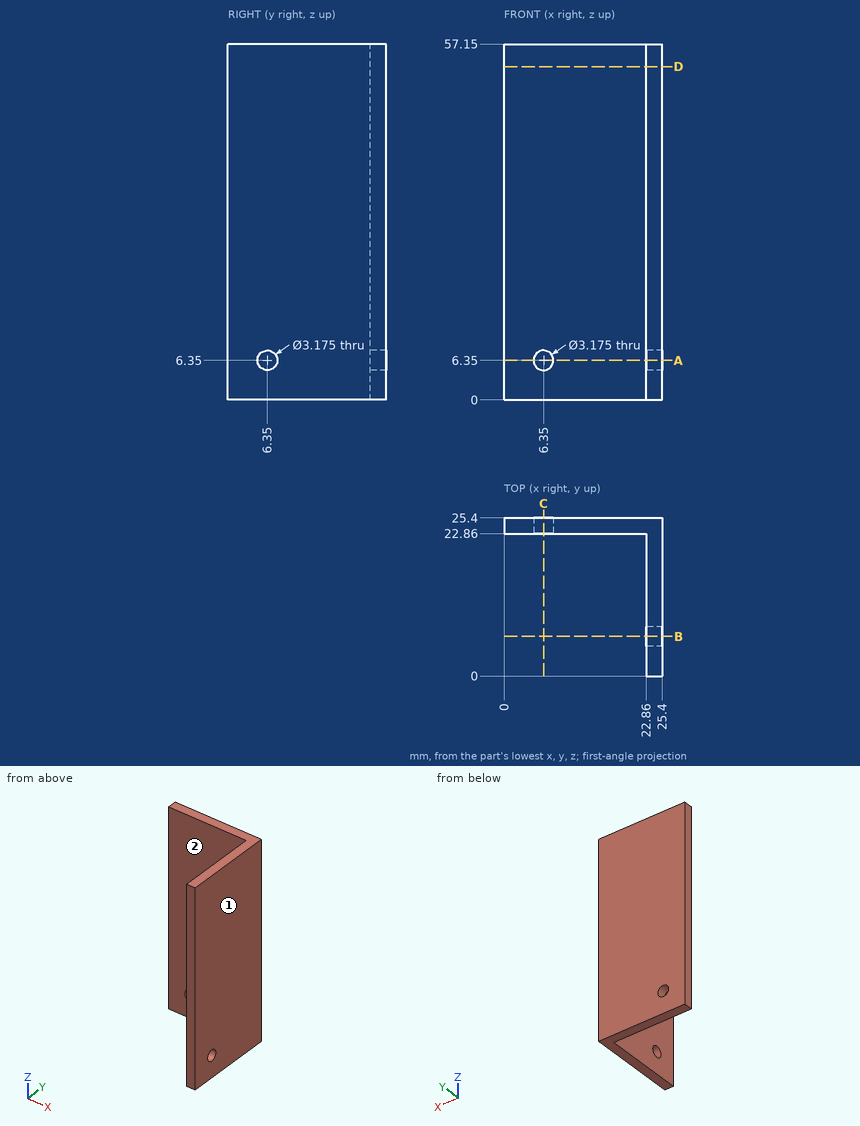
Job drawing, mm, ordinate dimensions from the low corner. One solid piece. A direction names the side the tool comes from. Give positions to 0.01 mm unless a question says otherwise; leave off trailing zeros. Write each loop counter-clockwise with the first axis right and the second up, starting at its lowest first coordinate (ties: lowest second). Pieces come first, ordered by that corner, then holes. Notation, with made-up numbers: M 22,-24 L 79,-24 A10 cw 79,-19 Z; hole C 72,27 d3. An arc over 180 degrees is marked long. Put each result on its own line as item: value. Start each with the question number.
(1) Flat gauge pins, fed straight in: pin 1 Ø3.5 at (x, z) = (6.35, 6.35) entering from -Y; pin 2 Ø10 at (y, z) = (11.5, 39) entering from -X; pin 3 Ø1.9 at (y, z) = (6.35, 6.35) entering from +X. Where does each tip first touch, or does it go through?
(2) Band-saw the part on D-D, the plane z = 53.5. Write the cut outline in (x, y), and give its area (3 significant figures).
(3) Which spindle directions (+Z, -Z, +X, -X, +Y, -Y) get a long thin tool onto all of the face, cutting with end or side? Do the marked faces 1 and 2. Say none if no direction does.
(4) Band-saw the part on B-B, the plane y = 6.35. Write the cut outline in (x, z), and give its area (3 significant figures).
(5) Probe L1, parallel to Z at x = 6.35, y = 23.55; L2, parallel to X at y = 14, z = 15.5. List the from-to ranges inside material, lowest first.
(6) Band-saw the part on A-A, the plane z = 6.35. Write the cut outline in (x, y).
Response values:
1. pin 1: stops at y = 22.86
1. pin 2: stops at x = 22.86
1. pin 3: passes through
2. outline: M 0,22.86 L 22.86,22.86 L 22.86,0 L 25.4,0 L 25.4,25.4 L 0,25.4 Z
2. area: 123 mm2
3. face 1: +Z, -Z, +X, +Y, -Y
3. face 2: +Z, -Z, -X, -Y
4. outline: M 22.86,0 L 25.4,0 L 25.4,4.76 L 22.86,4.76 Z; M 22.86,7.94 L 25.4,7.94 L 25.4,57.15 L 22.86,57.15 Z
4. area: 137 mm2
5. L1: z = 0 to 4.76, 7.94 to 57.15
5. L2: x = 22.86 to 25.4
6. outline: M 0,22.86 L 4.76,22.86 L 4.76,25.4 L 0,25.4 Z; M 7.94,22.86 L 22.86,22.86 L 22.86,7.94 L 25.4,7.94 L 25.4,25.4 L 7.94,25.4 Z; M 22.86,0 L 25.4,0 L 25.4,4.76 L 22.86,4.76 Z
